Design review of the part built by this model. Coordinates are the model's own, in mm. Face numbers are marked on the shaded views. A direction names the side the tool comes from. Coordinates: 2 decimals unless noted, no trailing zeros. Write each loop counter-clockwise with the first axis right and the second up, starting at its lowest first coordinate (ties: lowest second). Pieces come first, ordered by that corner, then holes. Notation, with made-up numbers: (34.25, 33) -> (41.25, 33) arc R20 cw to (41.25, 59) -> close; hole circle Ø3 at (-19.75, -34.5). An arc over 180 degrees is marked (long way). Answer in a Markdown table with one row per item. Add a question column.
Item 1: To check wall thickness, follow line 1 (X direction, y = 124.5, z = -205); line 2 (Z direction, x = 343, y = 300.5); line 3 (Y direction, x = -312.5, z = 634). State the ranges of each line that lie inside material, in increasing order.
Item 2: Take a section at C-C, the plane y = 137. Give the number of separate pieces and of enclosed holes in the cut face, and give its area (3 significant figures).
Item 3: Take a section at B-B, the plane x = 220. Write out the cut boundary in (y, z).
Item 4: Take a section at A-A, the plane z = -101. Write out the cut boundary in (x, y).
Item 5: Clearance check with a flat-ended pin moving along its axis: P1, Ø8, axis at x = 213.5, z = 596.5, coming from the -Y side. State where the tip first meets the part, or that it passes through.
Item 6: Draft analysis for pull direction Z (two halves, no side actions). For the marked faces 3, 4, 5 and 6, state which applies: released by +Z, released by -Z, zero draft, split by the parting line, or undercut.
Item 7: For the marked faces 1 and 2, list the 3-axis set-ups (+Z, -Z, +X, -X, +Y, -Y) from which the entire face can be reached by the end or side of a thin tool; tool diameter is ignored.
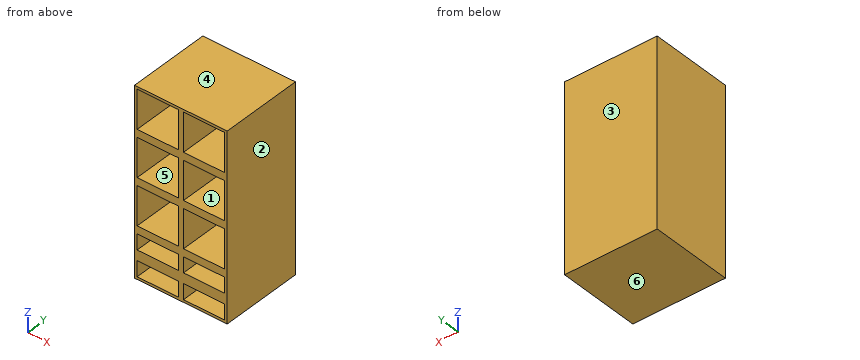
from build123d import *

# Parameters (mm, degrees)
F0_W     = 457.2
F0_H     = 1828.8
F1_DEPTH = 812.8
F2_W     = 406.4
F2_H     = 381
F2_H_2   = 152.4
F3_DEPTH = 457.2


with BuildPart() as f1:
    # F0 (on Front) → F1 (new body)
    with BuildSketch(Plane.XZ):
        with Locations((-228.6, 0)):
            Rectangle(F0_W, F0_H)
        with Locations((228.6, 0)):
            Rectangle(F0_W, F0_H)
    extrude(amount=-F1_DEPTH)

    # F2 (on face) → F3 (cut)
    with BuildSketch(Plane.XZ):
        with Locations((228.6, 698.5)):
            Rectangle(F2_W, F2_H)
        with Locations((228.6, 241.3)):
            Rectangle(F2_W, F2_H)
        with Locations((-228.6, 698.5)):
            Rectangle(F2_W, F2_H)
        with Locations((228.6, -215.9)):
            Rectangle(F2_W, F2_H)
        with Locations((-228.6, 241.3)):
            Rectangle(F2_W, F2_H)
        with Locations((228.6, -558.8)):
            Rectangle(F2_W, F2_H_2)
        with Locations((-228.6, -215.9)):
            Rectangle(F2_W, F2_H)
        with Locations((228.6, -812.8)):
            Rectangle(F2_W, F2_H_2)
        with Locations((-228.6, -558.8)):
            Rectangle(F2_W, F2_H_2)
        with Locations((-228.6, -812.8)):
            Rectangle(F2_W, F2_H_2)
    extrude(amount=-F3_DEPTH, mode=Mode.SUBTRACT)


solid = f1.part
Answers:
| question | item | result |
|---|---|---|
| 1 | line 1 | x = -457.2 to -431.8, -25.4 to 25.4, 431.8 to 457.2 |
| 1 | line 2 | z = -914.4 to -889, -736.6 to -635, -482.6 to -406.4, -25.4 to 50.8, 431.8 to 508, 889 to 914.4 |
| 1 | line 3 | y = 457.2 to 812.8 |
| 2 | separate pieces | 1 |
| 2 | enclosed holes | 10 |
| 2 | area | 495,000 mm^2 |
| 3 | outline | (0, -914.4) -> (812.8, -914.4) -> (812.8, 914.4) -> (0, 914.4) -> (0, 889) -> (457.2, 889) -> (457.2, 508) -> (0, 508) -> (0, 431.8) -> (457.2, 431.8) -> (457.2, 50.8) -> (0, 50.8) -> (0, -25.4) -> (457.2, -25.4) -> (457.2, -406.4) -> (0, -406.4) -> (0, -482.6) -> (457.2, -482.6) -> (457.2, -635) -> (0, -635) -> (0, -736.6) -> (457.2, -736.6) -> (457.2, -889) -> (0, -889) -> close |
| 4 | outline | (-457.2, 0) -> (-431.8, 0) -> (-431.8, 457.2) -> (-25.4, 457.2) -> (-25.4, 0) -> (25.4, 0) -> (25.4, 457.2) -> (431.8, 457.2) -> (431.8, 0) -> (457.2, 0) -> (457.2, 812.8) -> (-457.2, 812.8) -> close |
| 5 | P1 | stops at y = 457.2 |
| 6 | face 3 | zero draft |
| 6 | face 4 | released by +Z |
| 6 | face 5 | undercut |
| 6 | face 6 | released by -Z |
| 7 | face 1 | -Y |
| 7 | face 2 | +Z, -Z, +X, +Y, -Y |
